Here's how the part is built. I have some questions about the finished solid (model axes, mm). Round coordinates to 2 decimals unless told otherwise and drop trailing zeros. Loops run counter-clockwise (first coordinate to the right, second up) from the corner with the lowest first, then second, coordinate; pieces in that order, holes last. Notation, with made-up numbers: M -20.5,64.25 L -2.5,64.25 A16 ccw -2.5,80.25 Z; hole C -11,-5 d8. An arc over 180 degrees is marked long. Answer as a JSON object with one key per item and string values.
from build123d import *

# Parameters (mm, degrees)
F0_W     = 95.25
F0_H     = 76.2
F0_R     = 23.749
F1_DEPTH = 25.4
F2_DEPTH = 25.4


with BuildPart() as f1:
    # F0 (on Front) → F1 (new body)
    with BuildSketch(Plane.XZ):
        with Locations((10.760576, 0.456677)):
            Rectangle(F0_W, F0_H)
        with Locations((10.63576, 0)):
            Circle(F0_R, mode=Mode.SUBTRACT)
    extrude(amount=F1_DEPTH)

    # F0 (on Front) → F2 (cut)
    with BuildSketch(Plane.XZ):
        with Locations((10.760576, 0.456677)):
            Rectangle(F0_W, F0_H)
        with Locations((10.63576, 0)):
            Circle(F0_R, mode=Mode.SUBTRACT)
    extrude(amount=-F2_DEPTH, mode=Mode.SUBTRACT)


solid = f1.part
Item 1: Please list where these lines run through material, in increasing order: probe 1 along Z at (x, y) = (10.5, -19.5); probe 2 along Z at (x, y) = (3.5, -24); probe 3 along X at (y, z) = (-11.5, -5). Write a range as from..to.
Resolved:
{"probe 1": "-37.64..-23.75, 23.75..38.56", "probe 2": "-37.64..-22.65, 22.65..38.56", "probe 3": "-36.86..-12.58, 33.85..58.39"}
Item 2: If we mould it in two halves opening along Z, with no side actions, what happens to faces 1 (the face through (-6.87, -12.52, 16.05)), 2 (the face through (10, -13, 38.557)), 3 (the face through (10, -25.4, 26))? For each: pulls with the +Z half, pulls with the -Z half, needs draft (parallel to the pull), parting line crosses it, or undercut.
Resolved:
{"face 1": "undercut", "face 2": "pulls with the +Z half", "face 3": "needs draft"}
Item 3: I want a section at B-B, the plane x = 21.5. Please give me the cut outline in (y, z), then the cut area to 3 significant figures.
Resolved:
{"outline": "M -25.4,-37.64 L 0,-37.64 L 0,-21.12 L -25.4,-21.12 Z; M -25.4,21.12 L 0,21.12 L 0,38.56 L -25.4,38.56 Z", "area": "863 mm²"}
Item 4: I want a section at A-A, the plane z = 0. Please give me the cut outline in (x, y), then the cut area to 3 significant figures.
Resolved:
{"outline": "M -36.86,-25.4 L -13.11,-25.4 L -13.11,0 L -36.86,0 Z; M 34.38,-25.4 L 58.39,-25.4 L 58.39,0 L 34.38,0 Z", "area": "1,210 mm²"}
Item 5: I want a section at C-C, the plane y = -14.5. Please give me the cut outline in (x, z), then the cut area to 3 significant figures.
Resolved:
{"outline": "M -36.86,-37.64 L 58.39,-37.64 L 58.39,38.56 L -36.86,38.56 Z; hole C 10.64,0 d47.5", "area": "5,490 mm²"}
Item 6: I'm going to push a flat-ended pin straight in: pin 1 Ø1 at (x, z) = (27.5, -29) entering from +Y. Where does the tip first touch, or does it pass through?
Resolved:
{"pin 1": "y = 0"}
